```python
from build123d import *

# Parameters (mm, degrees)
SKETCH1_R           = 102.5
SKETCH1_R_2         = 100
BOSS_EXTRUDE1_DEPTH = 20
BOSS_EXTRUDE2_START = -10
BOSS_EXTRUDE2_DEPTH = 10
SKETCH3_W           = 20
SKETCH3_H           = 20
BOSS_EXTRUDE3_DEPTH = 44
BOSS_EXTRUDE5_DEPTH = 20


with BuildPart() as part:
    # Sketch1 → Boss-Extrude1 (new body)
    with BuildSketch(Plane(origin=(0, 0, 0), x_dir=(1, 0, 0), z_dir=(0, 1, 0))):
        with Locations(Location((0, 0, 0), (0, 0, 270))):
            Circle(SKETCH1_R)
        with Locations(Location((0, 0, 0), (0, 0, 270))):
            Circle(SKETCH1_R_2, mode=Mode.SUBTRACT)
    extrude(amount=BOSS_EXTRUDE1_DEPTH)

    # Sketch2 → Boss-Extrude2 (add)
    with BuildSketch(Plane(origin=(0, 20, 0), x_dir=(1, 0, 0), z_dir=(0, 1, 0)).offset(BOSS_EXTRUDE2_START)):
        with BuildLine():
            ThreePointArc((2.798561789, -102.461788253), (0.298650634, -102.499564915), (-2.201438211, -102.476356638))
            Line((-2.201438211, -102.476356638), (-2.201438211, -112.461788253))
            Line((-2.201438211, -112.461788253), (2.798561789, -112.461788253))
            Line((2.798561789, -112.461788253), (2.798561789, -102.461788253))
        make_face()
    extrude(amount=BOSS_EXTRUDE2_DEPTH)

    # Sketch3 → Boss-Extrude3 (add)
    with BuildSketch(Plane.XY.offset(112.461788253)):
        with Locations((0.298561789, 10)):
            Rectangle(SKETCH3_W, SKETCH3_H)
    extrude(amount=BOSS_EXTRUDE3_DEPTH)

    # Sketch4 → Boss-Extrude5 (add)
    with BuildSketch(Plane.ZY.offset(9.701438211)):
        with BuildLine():
            Line((145.311788254, 0), (139.711788253, 0))
            Line((139.711788253, 0), (139.711788253, -5.1))
            Line((139.711788253, -5.1), (140.211788253, -5.1))
            ThreePointArc((140.211788253, -5.1), (141.705543669, -1.493755415), (145.311788254, 0))
        make_face()
        with BuildLine():
            Line((150.911788253, 0), (145.311788254, 0))
            ThreePointArc((145.311788254, 0), (148.918032837, -1.493755416), (150.411788253, -5.1))
            Line((150.411788253, -5.1), (150.911788253, -5.1))
            Line((150.911788253, -5.1), (150.911788253, 0))
        make_face()
    extrude(amount=-BOSS_EXTRUDE5_DEPTH)


solid = part.part
```
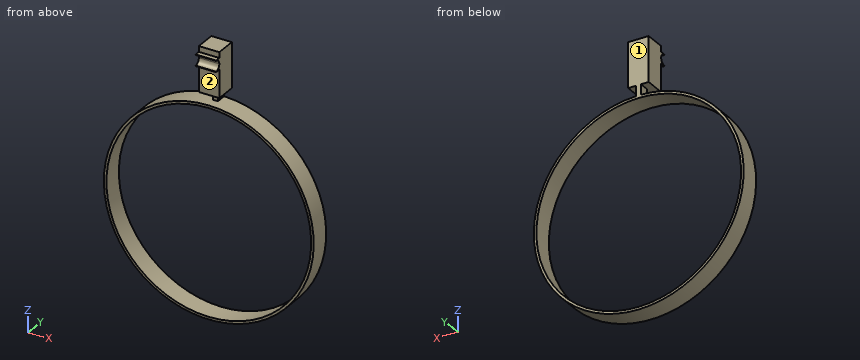
Geometry: final body of the model. Coordinates: model frame, mm. Face numbers are marked on the shaded views. A direction names the side the tool comes from. Coordinates: 2 decimals unless noted, no trailing zeros. Loops run counter-clockwise (first coordinate to the right, second up) from the corner with the lowest first, then second, coordinate; pieces in that order, holes last. Notation, with made-up numbers: M 82.25,41.25 L 87.25,41.25 A3 ccw 87.25,46.25 Z; hole C -35.75,23 d9. An arc over 180 degrees is marked long. Put each result on its own line as item: value.
(1) First-contact query: pin 1 (1 mm diameter, centred on x = -33, y = 12, fed in from +Z); pin 2 (1.5 mm diameter, centred on y = 12, z = -59, fed in from +X); pin 3 (12 mm diameter, centred on y = 17, z = -48.5, fed in from -X). Flat tips, straight axial feed; report the tip coordinate or a pass-through.
Answer sheet:
pin 1: stops at z = 97.21
pin 2: stops at x = 84.34
pin 3: stops at x = -93.27
(2) Cut plane C-C on x = -31. Return the cut outline in (y, z).
Answer sheet:
outline: M 0,-97.7 L 20,-97.7 L 20,-95.07 L 0,-95.07 Z; M 0,95.07 L 20,95.07 L 20,97.7 L 0,97.7 Z
(3) Cut plane B-B on z = 0. Return the cut outline in (x, y), then the cut area to 3 significant figures.
Answer sheet:
outline: M -102.5,0 L -100,0 L -100,20 L -102.5,20 Z; M 100,0 L 102.5,0 L 102.5,20 L 100,20 Z
area: 100 mm^2
(4) Material intervals for probe 1 along Z at (x, y) = (2, 4.5); probe 2 along X at (y, z) = (6, 0); probe 3 along Z at (x, y) = (-7.5, 10.25), sorted ascending.
Answer sheet:
probe 1: z = -102.48 to -99.98, 99.98 to 102.48, 112.46 to 156.46
probe 2: x = -102.5 to -100, 100 to 102.5
probe 3: z = -102.23 to -99.72, 99.72 to 102.23, 112.46 to 156.46
(5) Access query for the marked faces 1 and 2. Directions: +Z, -Z, +X, -X, +Y, -Y. A direction counts if a zero-diameter tool reaches every point of the face in a straight line with its end or side. Return the directions, or none.
Answer sheet:
face 1: +Z, -Z, +X, -X, +Y
face 2: -Z, +X, -X, -Y
(6) Cut plane D-D on z = 129. Return the cut outline in (x, y).
Answer sheet:
outline: M -9.7,0 L 10.3,0 L 10.3,20 L -9.7,20 Z
(7) Cut plane A-A on y = 6.25. Return the cut outline in (x, z).
Answer sheet:
outline: C 0,0 d205; M -9.7,112.46 L 10.3,112.46 L 10.3,156.46 L -9.7,156.46 Z; hole C 0,0 d200
